Could you check a few things on this model? Use its own coordinates, in mm. A direction names the side the tool comes from. Coordinates: 2 decimals unless noted, no trailing zeros. Loops run counter-clockwise (first coordinate to the right, second up) from the corner with the lowest first, then second, coordinate; pieces in that order, holes last. Notation, with made-up numbers: (2.5, 79.5) -> (20.5, 79.5) arc R35 cw to (20.5, 112.5) -> close; hole circle Ø10 at (74, 10). An arc over 180 degrees is marked (long way). One line per question, with ' | ' between items.
```python
from build123d import *

# Parameters (mm, degrees)
FILLET1_R         = 2
CHAMFER1_SIZE     = 1
CIRPATTERN1_COUNT = 4


with BuildPart() as part:
    # Sketch1 → Revolve1 (revolve)
    with BuildSketch(Plane.XY):
        Polygon((-32.5, 42.5), (32.5, 42.5), (32.5, 31), (-28.5, 31), (-28.5, 28.5), (-32.5, 28.5), align=None)
    revolve(axis=Axis((88.99, 0, 0), (-1, 0, 0)))

    # Fillet1
    fillet1_edges = [part.edges().sort_by_distance(p)[0] for p in [
        (-32.5, -42.5, 0),
    ]]
    fillet(fillet1_edges, radius=FILLET1_R)

    # Chamfer1
    chamfer1_edges = [part.edges().sort_by_distance(p)[0] for p in [
        (-32.5, -28.5, 0),
    ]]
    chamfer(chamfer1_edges, length=CHAMFER1_SIZE)

    # Sketch5 → Tap Drill for M5x0.8 Tap1 (revolve, cut)
    with BuildSketch(Plane(origin=(32.5, 37, 0), x_dir=(0, 0, -1), z_dir=(0, 1, 0))):
        Polygon((0, 0), (0, 21.2618073), (2.1, 20), (2.1, 0), align=None)
    tap_drill_for_m5x0_8_tap1 = revolve(axis=Axis((38.85, 37, 0), (-1, 0, 0)), mode=Mode.SUBTRACT)

    # CirPattern1: Tap Drill for M5x0.8 Tap1 ×4 about axis
    cirpattern1_axis = Axis((0, 0, 0), (1, 0, 0))
    for i in range(1, CIRPATTERN1_COUNT):
        add(tap_drill_for_m5x0_8_tap1.rotate(cirpattern1_axis, i * 360 / CIRPATTERN1_COUNT), mode=Mode.SUBTRACT)


solid = part.part
```
Q1. Please list where these lines run through material, in increasing order: L1, parallel to Z at x = 27.25, y = 0; L2, parallel to Z at x = -30.1, y = 0; L3, parallel to Z at x = 4, y = -1. Write a range as [from, to].
Values follow:
L1: z = [-42.5, -39.1], [-34.9, -31], [31, 34.9], [39.1, 42.5] | L2: z = [-42.5, -28.5], [28.5, 42.5] | L3: z = [-42.49, -30.98], [30.98, 42.49]
Q2. For pin 1 (1.5 mm diameter, centred on x = -11, z = -21, fed in from -Y); pin 2 (1 mm diameter, centred on x = 11, z = 27.5, fed in from -Y); pin 3 (12 mm diameter, centred on x = -10, z = -28.5, fed in from -Y), each with a flat end and sliding along its axis, tell me the tip position at first contact or that it passes through.
Values follow:
pin 1: stops at y = -37.37 | pin 2: stops at y = -32.82 | pin 3: stops at y = -36.06
Q3. We'd pull the mould along Z, two halves only. Please class faces 1 (the face through (1.441, -33.727, 25.861)), 2 (the face through (32.5, -22.24, 21.84)), 3 (the face through (11.46, 0.2, 36.69)), 4 (the face through (22.64, -39.05, -0.46)): released by +Z, released by -Z, zero draft, split by the parting line, or undercut.
Values follow:
face 1: split by the parting line | face 2: zero draft | face 3: undercut | face 4: undercut
Q4. For faces 5 (the face through (22.64, 39.05, 0.46)), 6 (the face through (-32.5, -3, 30)), which set-ups out of +Z, -Z, +X, -X, +Y, -Y let a thin tool reach every point of the face, with its end or its side?
Values follow:
face 5: +X | face 6: +Z, -Z, -X, +Y, -Y
Q5. Imagine slicing it at A-A on x = 22. Write out the boundary of the cut face in (y, z).
Values follow:
outline: circle Ø85 at (0, 0); hole circle Ø4.2 at (-37, 0); hole circle Ø62 at (0, 0); hole circle Ø4.2 at (0, -37); hole circle Ø4.2 at (0, 37); hole circle Ø4.2 at (37, 0)
